```python
from build123d import *

# Parameters (mm, degrees)
SKETCH1_W           = 1000
SKETCH1_H           = 1600
SKETCH1_W_2         = 940
SKETCH1_H_2         = 1540
BOSS_EXTRUDE1_DEPTH = 15
SKETCH2_W           = 26
SKETCH2_H           = 26


with BuildPart() as part:
    # Sketch1 → Boss-Extrude1 (new body, symmetric)
    with BuildSketch(Plane.XY):
        Rectangle(SKETCH1_W, SKETCH1_H)
        Rectangle(SKETCH1_W_2, SKETCH1_H_2, mode=Mode.SUBTRACT)
    extrude(amount=BOSS_EXTRUDE1_DEPTH, both=True)

    # Cut-Sweep1: sweep along a path in Sketch4
    with BuildLine(Plane.XY) as cut_sweep1_path:
        Line((-485, 785), (-485, -785))
        Line((-485, -785), (485, -785))
        Line((485, -785), (485, 785))
        Line((485, 785), (-485, 785))
    # Sketch2 → Cut-Sweep1 (sweep, cut)
    with BuildSketch(Plane(origin=(0, 0, 0), x_dir=(0, 0, -1), z_dir=(1, 0, 0))):
        with Locations((0, 785)):
            Rectangle(SKETCH2_W, SKETCH2_H)
    sweep(path=cut_sweep1_path.line, transition=Transition.RIGHT, mode=Mode.SUBTRACT)

    # Sketch7 → Revolve1 (revolve)
    with BuildSketch(Plane.XY):
        with BuildLine():
            Line((-340, 800), (-340, 805))
            Line((-340, 805), (-345, 805))
            ThreePointArc((-345, 805), (-342.5, 802.5), (-345, 800))
            Line((-345, 800), (-340, 800))
        make_face()
    revolve1 = revolve(axis=Axis((-340, 795.104340353, 0), (0, 1, 0)))

    # Mirror1: Revolve1 across plane
    add(revolve1.mirror(Plane(origin=(0, 0, 0), x_dir=(0, 0, 1), z_dir=(1, 0, 0))))


solid = part.part
```
The model under review builds one solid part; all positions refer to its coordinate system, in mm. A direction names the side the tool comes from. Round coordinates to 2 decimals unless told otherwise and drop trailing zeros. Loops run counter-clockwise (first coordinate to the right, second up) from the corner with the lowest first, then second, coordinate; pieces in that order, holes last.
1) Wall thickness on line 1 along X through (y, z) = (-546, -5.25); line 2 along Y through (x, z) = (5.5, 1.75); line 3 along X through (y, z) = (516, 13.5): over which ranges is each line inside the solid? List them lowest first.
Values follow:
line 1: x = -500 to -498, -472 to -470, 470 to 472, 498 to 500
line 2: y = -800 to -798, -772 to -770, 770 to 772, 798 to 800
line 3: x = -500 to -470, 470 to 500
2) Consider section B-B on y = -333. State the section outline as (x, z) points.
Values follow:
outline: (-500, -15) - (-470, -15) - (-470, 15) - (-500, 15) - close; (470, -15) - (500, -15) - (500, 15) - (470, 15) - close; hole (-498, -13) - (-472, -13) - (-472, 13) - (-498, 13) - close; hole (472, -13) - (498, -13) - (498, 13) - (472, 13) - close
3) The part is to be moulded in two halves that separate along Y. For faces 1 (the face through (-7, -800, 0)), 2 (the face through (-7, 800, 0)), 3 (the face through (500, -11, 0)), 4 (the face through (-470, -11, 0)), say which applies: pulls with the +Y half, pulls with the -Y half, needs draft (parallel to the pull), parting line crosses it, or undercut.
Values follow:
face 1: pulls with the -Y half
face 2: pulls with the +Y half
face 3: needs draft
face 4: undercut
4) Consider section A-A on x = -204. State the section outline as (y, z) points.
Values follow:
outline: (-800, -15) - (-770, -15) - (-770, 15) - (-800, 15) - close; (770, -15) - (800, -15) - (800, 15) - (770, 15) - close; hole (-798, -13) - (-772, -13) - (-772, 13) - (-798, 13) - close; hole (772, -13) - (798, -13) - (798, 13) - (772, 13) - close
5) Tool access review of faces 5 (the face through (-484, 241, 15)), 6 (the face through (-477, -240, -13)), 7 (the face through (-7, 770, 0)): name each direction out of +Z, -Z, +X, -X, +Y, -Y from which nothing blocks a thin tool from reaching the whole face with its end or side.
Values follow:
face 5: +Z, +X, -X, +Y, -Y
face 6: none
face 7: +Z, -Z
6) Clearance check with a flat-ended pin moving along its axis: P1, Ø13, axis at x = 217, z = -6.5, coming from the +Y side. State where the tip first meets the part, or that it passes through.
Values follow:
P1: stops at y = 800
